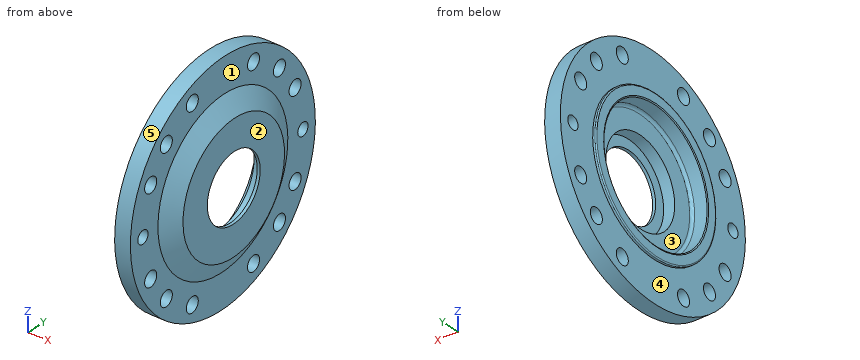
from build123d import *

# Parameters (mm, degrees)
ESQUISSE2_R             = 7
ESQUISSE2_R_2           = 5.983
ENL_V_MAT_EXTRU_1_DEPTH = 154.98944769
ESQUISSE3_R             = 30.75
ENL_V_MAT_EXTRU_2_DEPTH = 153.723114362
CONG_2_R                = 1
CONG_3_R                = 2.5


with BuildPart() as part:
    # Esquisse1 → Révolution1 (revolve)
    with BuildSketch(Plane.XY, mode=Mode.PRIVATE) as r_volution1_sk:
        Polygon((85.536385131, 40), (85.536385131, 0), (88.292789625, 0), (88.292789625, 59), (78.292789625, 75.5), (78.292789625, 107.5), (63.792789625, 107.5), (63.792789625, 70), (60.792789625, 70), (60.792789625, 61), (61.398850231, 60), (75.347845805, 60), (75.347845805, 40), align=None)
    revolve(r_volution1_sk.sketch.rotate(Axis((85.536385131, 0, 0), (1, 0, 0)), 90), axis=Axis((85.536385131, 0, 0), (1, 0, 0)))

    # Esquisse2 → Enlèv. mat.-Extru.1 (cut, through all)
    with BuildSketch(Plane.ZY.offset(-63.792789625)):
        with Locations((-40.037532003, 83.940431445)):
            Circle(ESQUISSE2_R)
        with Locations((-65.76093065, 65.76093065)):
            Circle(ESQUISSE2_R)
        with Locations((-85.920796524, 35.58955921)):
            Circle(ESQUISSE2_R)
        with Locations((40.037532003, 83.940431445)):
            Circle(ESQUISSE2_R)
        with Locations((65.76093065, 65.76093065)):
            Circle(ESQUISSE2_R)
        with Locations((85.920796524, 35.58955921)):
            Circle(ESQUISSE2_R)
        with Locations((85.920796524, -35.58955921)):
            Circle(ESQUISSE2_R)
        with Locations((65.76093065, -65.76093065)):
            Circle(ESQUISSE2_R)
        with Locations((40.037532003, -83.940431445)):
            Circle(ESQUISSE2_R)
        with Locations((-40.037532003, -83.940431445)):
            Circle(ESQUISSE2_R)
        with Locations((-65.76093065, -65.76093065)):
            Circle(ESQUISSE2_R)
        with Locations((-85.920796524, -35.58955921)):
            Circle(ESQUISSE2_R)
        with Locations((0, 93)):
            Circle(ESQUISSE2_R_2)
        with Locations((0, -93)):
            Circle(ESQUISSE2_R_2)
    extrude(amount=-ENL_V_MAT_EXTRU_1_DEPTH, mode=Mode.SUBTRACT)

    # Esquisse3 → Enlèv. mat.-Extru.2 (cut, through all)
    with BuildSketch(Plane.ZY.offset(-75.347845805)):
        Circle(ESQUISSE3_R)
    extrude(amount=-ENL_V_MAT_EXTRU_2_DEPTH, mode=Mode.SUBTRACT)

    # Congé2
    cong_2_edges = [part.edges().sort_by_distance(p)[0] for p in [
        (60.792789625, 0, -70),
    ]]
    fillet(cong_2_edges, radius=CONG_2_R)

    # Congé3
    cong_3_edges = [part.edges().sort_by_distance(p)[0] for p in [
        (75.347845805, 0, -60),
    ]]
    fillet(cong_3_edges, radius=CONG_3_R)


solid = part.part
Can you work these out from the model? Positions are in its coordinate system, mm. Face numbers are marked on the shaded views. A direction names the side the tool comes from. Coordinates: 2 decimals unless noted, no trailing zeros. Order: outer loops, then holes, each group sorted by start corner. A loop starts at its lowest first (then second) coordinate and runs counter-clockwise, first axis right, second up. Notation, with made-up numbers: M -29,86.5 L 18,86.5 A22 ccw 18,122.5 Z; hole C -10.5,9 d8. An arc over 180 degrees is marked long. Write item = value, one per line.
(1) Suppose I cut it at B-B on x = 68.25. State how many separate pieces and enclosed holes the cut face has, plus the area to 3 significant figures.
Results are:
separate_pieces = 1
enclosed_holes = 15
area = 22,900 mm2
(2) Suppose I cut it at C-C on z = -89.5. Please give me the cut outline in (x, y), plus the area to 3 significant figures.
Results are:
outline = M 63.79,-59.55 L 78.29,-59.55 L 78.29,-41.61 L 63.79,-41.61 Z; M 63.79,-29.57 L 78.29,-29.57 L 78.29,29.57 L 63.79,29.57 Z; M 63.79,41.61 L 78.29,41.61 L 78.29,59.55 L 63.79,59.55 Z
area = 1,380 mm2
(3) For the marked faces 1 and 2, which set-ups out of +Z, -Z, +X, -X, +Y, -Y let a thin tool reach every point of the face, with its end or its side?
Results are:
face_1 = +X
face_2 = +Z, -Z, +X, +Y, -Y
(4) If we mould it in two halves opening along Y, with no side actions, what happens to the marked faces 3, 4 and 5? For each: pulls with the +Y half, pulls with the -Y half, needs draft (parallel to the pull), parting line crosses it, or undercut.
Results are:
face_3 = undercut
face_4 = needs draft
face_5 = parting line crosses it
(5) I need wall thicknesses on line 1 along Y through (x, z) = (69.25, 0); line 2 along Z through (x, y) = (69, 82); line 3 along Y through (x, z) = (74, -76.5). Which ranges of each line are inside material? Lowest first, please. Write a range as [from, to].
Results are:
line_1 = [-107.5, -98.98], [-87.02, -60], [60, 87.02], [98.98, 107.5]
line_2 = [-69.51, -46.76], [-33.31, 33.31], [46.76, 69.51]
line_3 = [-75.52, 75.52]
(6) For pin 1 Ø5 at (x, z) = (64.5, 78.5) entering from +Y; pin 2 Ø16 at (y, z) = (-83.94, 40.04) entering from +X; pin 3 Ø22.5 at (y, z) = (-35.59, 85.92) entering from -X, each with a flat end and sliding along its axis, tell me the tip position at first contact or that it passes through.
Results are:
pin_1 = 76.03
pin_2 = 78.29
pin_3 = 63.79
